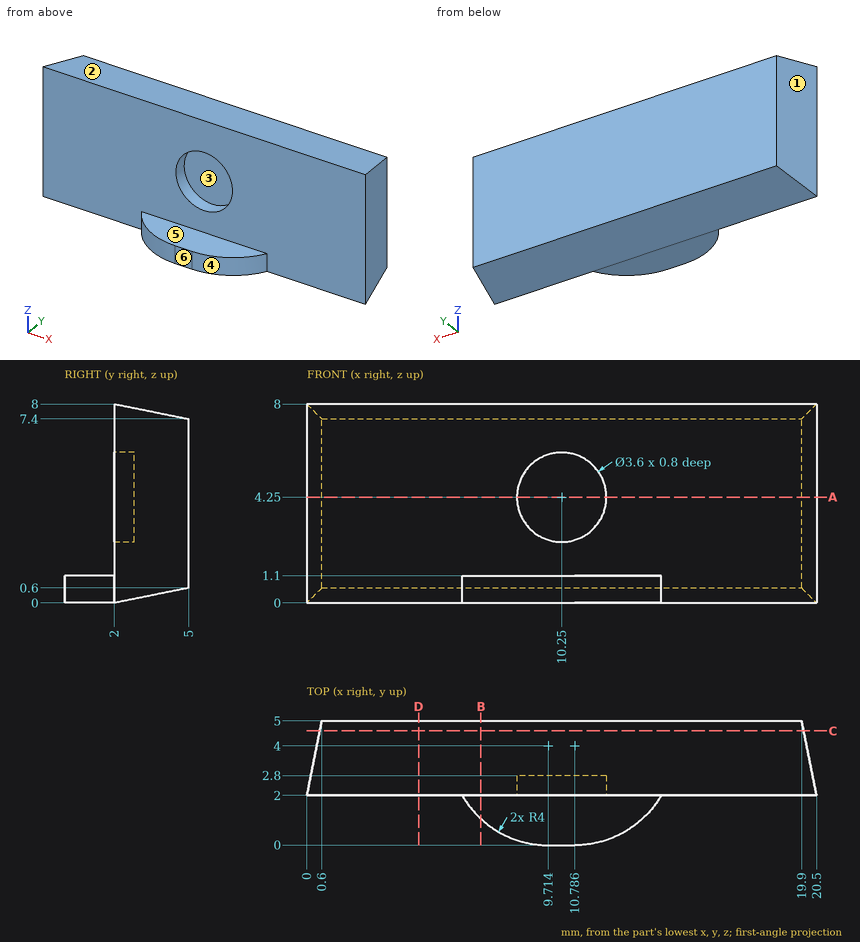
Print and shaded views of the part. All mm, measured from the part's lowest x, y and z. A direction names the side the tool comes from. Give positions to 0.01 mm unless a question says otherwise; leave off trailing zeros. Write each loop counter-clockwise with the first axis right and the second up, starting at its lowest first coordinate (ties: lowest second). Pieces come first, ordered by that corner, then holes. Notation, with made-up numbers: (1, -19) -> (19, -19) arc R26 ccw to (19, 9) -> close; hole circle Ø5 at (6.5, 10.25). An arc over 180 degrees is marked (long way). Use CSV: the item, a comma, the result in double quotes. Start each with the question number.
1) Two-plate mould, pull along X, no slides. Class the marked faces 1, 2, 3 and 4: released by +X, released by -X, zero draft, split by the parting line, or undercut.
2) Pin check, flat tips, straight feed: P1, Ø2.5, axis at x = 12, z = 5, coming from the -Y side; P2, Ø2, axis at x = 12.5, y = 4, coming from the -Z side; P3, Ø1.8, axis at x = 9.5, z = 4.5, coming from the -Y side. Stop position of each tip, or through.
3) Cut at A-A on z = 4.25. List the corners of the cut face in (x, y).
4) Cut at C-C on y = 4.6. List the corners of the cut face in (x, z).
5) Cut at B-B on x = 7. List the corners of the cut face in (y, z).
6) Drill centre lines: L1, parallel to Y at x = 17.5, z = 7; L2, parallel to Y at x = 9, z = 4; L3, parallel to X at y = 2.65, z = 4.25. Where is each one in solid material? Low to high.
7) Cut at D-D on x = 4.5. List the corners of the cut face in (y, z), plus the area to 3 significant figures.
8) Tool access for the marked faces 5 and 6: list every direction of +Z, -Z, +X, -X, +Y, -Y with a clear straight run to the whole face (end or side of a thin tool).
Final values:
1,face 1,"released by -X"
1,face 2,"zero draft"
1,face 3,"undercut"
1,face 4,"released by +X"
2,P1,"stops at y = 2"
2,P2,"stops at z = 0.2"
2,P3,"stops at y = 2.8"
3,outline,"(0, 2) -> (8.45, 2) -> (8.45, 2.8) -> (12.05, 2.8) -> (12.05, 2) -> (20.5, 2) -> (19.9, 5) -> (0.6, 5) -> close"
4,outline,"(0.52, 0.52) -> (19.98, 0.52) -> (19.98, 7.48) -> (0.52, 7.48) -> close"
5,outline,"(1.06, 0) -> (2, 0) -> (5, 0.6) -> (5, 7.4) -> (2, 8) -> (2, 1.1) -> (1.06, 1.1) -> close"
6,L1,"y = 2 to 5"
6,L2,"y = 2.8 to 5"
6,L3,"x = 0.13 to 8.45, 12.05 to 20.37"
7,outline,"(2, 0) -> (5, 0.6) -> (5, 7.4) -> (2, 8) -> close"
7,area,"22.2 mm2"
8,face 5,"+Z, +X, -X, -Y"
8,face 6,"+Z, -Z, +X, -X, -Y"
